Could you check a few things on this model? Use its own coordinates, in mm. Face numbers are marked on the shaded views. A direction names the side the tool comes from. Round coordinates to 2 decimals unless told otherwise and drop trailing zeros. Loops run counter-clockwise (first coordinate to the right, second up) from the corner with the lowest first, then second, coordinate; pieces in that order, holes last. Notation, with made-up numbers: M 44,-9.5 L 91,-9.5 A16 ccw 91,3.5 Z; hole C 18,18 d6. An arc over 180 degrees is marked long. Return JSON: item names as keys, results as strings. Group by question number.
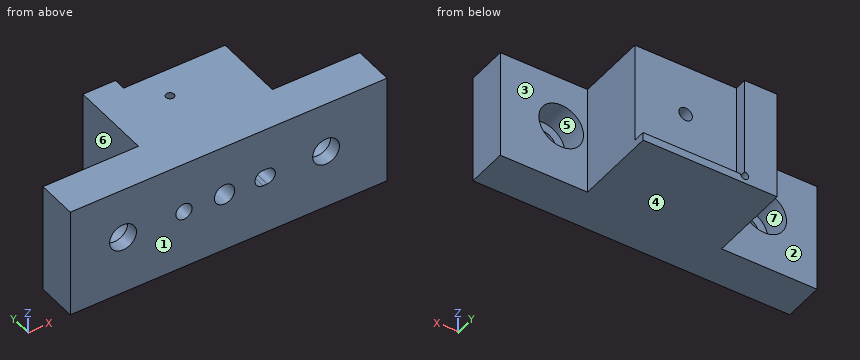
```python
from build123d import *

# Parameters (mm, degrees)
SKETCH_1_W                = 29
SKETCH_1_H                = 29
EXTRUDE_1_DEPTH           = 5
SKETCH_2_W                = 25
SKETCH_2_H                = 25
CUT_EXTRUDE_1_DEPTH       = 3
SKETCH_3_W                = 35
SKETCH_3_H                = 29
EXTRUDE_748_DEPTH         = 25.341167732
HOLE_WIZARD_M4_1_D        = 3.3
HOLE_WIZARD_M4_1_DEPTH    = 10.1
HOLE_WIZARD_M4_1_TIP      = 0.991420021
SKETCH_9_R                = 1
CUT_EXTRUDE_2_DEPTH       = 3
SKETCH_11_W               = 29
SKETCH_11_H               = 5
EXTRUDE_4_DEPTH           = 6
CUT_EXTRUDE_8_DEPTH       = 40.383835
SKETCH_19_W               = 80
SKETCH_19_H               = 25
EXTRUDE_5_DEPTH           = 10
HOLE_WIZARD_1_D           = 6.6
HOLE_WIZARD_1_DEPTH       = 10.1
HOLE_WIZARD_1_CBORE_D     = 11
HOLE_WIZARD_1_CBORE_DEPTH = 6.8
HOLE_WIZARD_1_TIP         = 1.982840043
SKETCH_23_W               = 80
SKETCH_23_H               = 10
EXTRUDE_6_DEPTH           = 2
SKETCH_24_W               = 27
SKETCH_24_H               = 10
CUT_EXTRUDE_9_DEPTH       = 2
MM_1_D                    = 4
MM_1_DEPTH                = 5
MM_1_TIP                  = 1.201721238
CUT_EXTRUDE_10_DEPTH      = 5
SKETCH_28_R               = 1
CUT_EXTRUDE_11_DEPTH      = 2
HOLE_WIZARD_M6_1_D        = 5
HOLE_WIZARD_M6_1_DEPTH    = 10
HOLE_WIZARD_M6_1_TIP      = 1.502151548


with BuildPart() as part:
    # 草图1 → 凸台-拉伸1 (new body)
    with BuildSketch(Plane(origin=(0, 0, 0), x_dir=(1, 0, 0), z_dir=(0, 1, 0))):
        Rectangle(SKETCH_1_W, SKETCH_1_H)
    extrude(amount=EXTRUDE_1_DEPTH)

    # 草图2 → 切除-拉伸1 (cut)
    with BuildSketch(Plane.XZ.offset(-5)):
        Rectangle(SKETCH_2_W, SKETCH_2_H)
    extrude(amount=CUT_EXTRUDE_1_DEPTH, mode=Mode.SUBTRACT)

    # 草图3 → Extrude 748 (add)
    with BuildSketch(Plane(origin=(0, 0, 0), x_dir=(-1, 0, 0), z_dir=(0, -1, 0))):
        with Locations((3, 0)):
            Rectangle(SKETCH_3_W, SKETCH_3_H)
    extrude(amount=EXTRUDE_748_DEPTH)

    # M4 螺纹孔1
    with Locations(Plane.ZX.offset(2)):
        with Locations((0, 0)):
            Hole(HOLE_WIZARD_M4_1_D / 2, depth=HOLE_WIZARD_M4_1_DEPTH)
            with Locations((0, 0, -(HOLE_WIZARD_M4_1_DEPTH + HOLE_WIZARD_M4_1_TIP / 2))):  # 118° drill point
                Cone(0, HOLE_WIZARD_M4_1_D / 2, HOLE_WIZARD_M4_1_TIP, mode=Mode.SUBTRACT)

    # 草图9 → 切除-拉伸2 (cut)
    with BuildSketch(Plane(origin=(0, 5, 0), x_dir=(1, 0, 0), z_dir=(0, 1, 0))):
        with Locations((-12.5, 12.5)):
            Circle(SKETCH_9_R)
    extrude(amount=-CUT_EXTRUDE_2_DEPTH, mode=Mode.SUBTRACT)

    # 草图11 → 凸台-拉伸4 (add)
    with BuildSketch(Plane.ZY.offset(14.5)):
        with Locations((0, 2.5)):
            Rectangle(SKETCH_11_W, SKETCH_11_H)
    extrude(amount=EXTRUDE_4_DEPTH)

    # 草图17 → 切除-拉伸8 (cut, through all)
    with BuildSketch(Plane(origin=(0, 5, 0), x_dir=(1, 0, 0), z_dir=(0, 1, 0))):
        Polygon((-20.5, -14.5), (14.5, -14.5), (14.5, 14.5), (12.5, 14.5), (12.5, -12.5), (-20.5, -12.5), align=None)
    extrude(amount=-CUT_EXTRUDE_8_DEPTH, mode=Mode.SUBTRACT)

    # 草图19 → 凸台-拉伸5 (add)
    with BuildSketch(Plane(origin=(0, -25.341167732, 0), x_dir=(-1, 0, 0), z_dir=(0, -1, 0))):
        with Locations((6, 0)):
            Rectangle(SKETCH_19_W, SKETCH_19_H)
    extrude(amount=-EXTRUDE_5_DEPTH)

    # 打孔尺寸(%根据)内六角圆柱头螺钉的类型1
    with Locations(Plane(origin=(-31, -15.341167732, 0), x_dir=(0, 0, 1), z_dir=(0, 1, 0))):
        with Locations((0, 0), (0, 50)):
            CounterBoreHole(HOLE_WIZARD_1_D / 2, HOLE_WIZARD_1_CBORE_D / 2, HOLE_WIZARD_1_CBORE_DEPTH, depth=HOLE_WIZARD_1_DEPTH)
            with Locations((0, 0, -(HOLE_WIZARD_1_DEPTH + HOLE_WIZARD_1_TIP / 2))):  # 118° drill point
                Cone(0, HOLE_WIZARD_1_D / 2, HOLE_WIZARD_1_TIP, mode=Mode.SUBTRACT)

    # 草图23 → 凸台-拉伸6 (add)
    with BuildSketch(Plane(origin=(0, 0, -12.5), x_dir=(-1, 0, 0), z_dir=(0, 0, -1))):
        with Locations((6, -20.341167732)):
            Rectangle(SKETCH_23_W, SKETCH_23_H)
    extrude(amount=EXTRUDE_6_DEPTH)

    # 草图24 → 切除-拉伸9 (cut)
    with BuildSketch(Plane.ZY.offset(46)):
        with Locations((-1, -20.341167732)):
            Rectangle(SKETCH_24_W, SKETCH_24_H)
    extrude(amount=-CUT_EXTRUDE_9_DEPTH, mode=Mode.SUBTRACT)

    # 大小mm 暗销孔1
    with Locations(Plane(origin=(-16, -25.341167732, 0), x_dir=(0, 0, -1), z_dir=(0, -1, 0))):
        with Locations((0, 0)):
            Hole(MM_1_D / 2, depth=MM_1_DEPTH)
            with Locations((0, 0, -(MM_1_DEPTH + MM_1_TIP / 2))):  # 118° drill point
                Cone(0, MM_1_D / 2, MM_1_TIP, mode=Mode.SUBTRACT)

    # 草图27 → 切除-拉伸10 (cut)
    with BuildSketch(Plane.XZ.offset(25.341167732)):
        with BuildLine():
            Line((3.5, 2), (4.5, 2))
            ThreePointArc((4.5, 2), (6.5, 0), (4.5, -2))
            Line((4.5, -2), (3.5, -2))
            ThreePointArc((3.5, -2), (1.5, 0), (3.5, 2))
        make_face()
    extrude(amount=-CUT_EXTRUDE_10_DEPTH, mode=Mode.SUBTRACT)

    # 草图28 → 切除-拉伸11 (cut)
    with BuildSketch(Plane.XY.offset(12.5)):
        with Locations((-6, -5.341167732)):
            Circle(SKETCH_28_R)
    extrude(amount=-CUT_EXTRUDE_11_DEPTH, mode=Mode.SUBTRACT)

    # M6 螺纹孔1
    with Locations(Plane(origin=(-6, -25.341167732, 0), x_dir=(0, 0, -1), z_dir=(0, -1, 0))):
        with Locations((0, 0)):
            Hole(HOLE_WIZARD_M6_1_D / 2, depth=HOLE_WIZARD_M6_1_DEPTH)
            with Locations((0, 0, -(HOLE_WIZARD_M6_1_DEPTH + HOLE_WIZARD_M6_1_TIP / 2))):  # 118° drill point
                Cone(0, HOLE_WIZARD_M6_1_D / 2, HOLE_WIZARD_M6_1_TIP, mode=Mode.SUBTRACT)


solid = part.part
```
1. I need wall thicknesses on probe 1 along X at (y, z) = (-16.75, 0); probe 2 along X at (y, z) = (-24.55, 0); probe 3 along Y at (x, z) = (21.5, 6.25). Which ranges of each line are inside material? Lowest first, please.
2. We'd pull the mould along Z, two halves only. Please class the marked faces 4, 5, 6 and 7: +Z half, -Z half, draft (parallel to the pull), parting line (faces both ways), or undercut.
3. If we section it at B-B, the plane z = 6.75: Please give me the cut outline in (x, y).
4. I'm going to push flat-ended pins straight in: pin 1 Ø10 at (y, z) = (-4.5, -5) entering from -X; pin 2 Ø9 at (x, z) = (-31, 0) entering from +Y; pin 3 Ø12 at (y, z) = (-9.5, 2) entering from -X; pin 4 Ø1.2 at (x, z) = (-12.5, -12.5) entering from +Y. Where does each tip first touch, or does it pass through?
5. If we section it at A-A, the plane y = 1: Please give me the cut outline in (x, z), then the cut area to 3 significant figures.
6. If we section it at C-C, the plane x = 2.5: Please give me the cut outline in (y, z), then the cut area to 3 significant figures.
7. On a 3-axis mill with a long thin cutter (end or side, diameter ignored), from which of +Z, -Z, +X, -X, +Y, -Y can I reach the whole of each face in a straight line? I mean the marked faces 1, 2 and 3. Say none if no direction works.
8. If we section it at D-D, the plane y = -11: Please give me the cut outline in (x, z).
Geometry results:
{
 "1": {"probe 1": "-44 to -36.5, -25.5 to -8.5, -3.5 to 13.5, 24.5 to 34", "probe 2": "-44 to -34.3, -27.7 to -18, -14 to -8.5, -3.5 to 1.5, 6.5 to 15.7, 22.3 to 34", "probe 3": "-25.34 to -15.34"},
 "2": {"face 4": "-Z half", "face 5": "undercut", "face 6": "draft", "face 7": "undercut"},
 "3": {"outline": "M -44,-25.34 L 34,-25.34 L 34,-15.34 L 12.5,-15.34 L 12.5,2 L -12.5,2 L -12.5,5 L -20.5,5 L -20.5,-15.34 L -44,-15.34 Z"},
 "4": {"pin 1": "x = -20.5", "pin 2": "y = -22.14", "pin 3": "x = -44", "pin 4": "y = 2"},
 "5": {"outline": "M -20.5,-14.5 L 12.5,-14.5 L 12.5,12.5 L -20.5,12.5 Z; hole C 0,0 d3.3", "area": "882 mm^2"},
 "6": {"outline": "M -25.34,-14.5 L 5,-14.5 L 5,-12.5 L 2,-12.5 L 2,12.5 L -25.34,12.5 L -25.34,1.73 L -20.34,1.73 L -20.34,-1.73 L -25.34,-1.73 Z", "area": "727 mm^2"},
 "7": {"face 1": "+Z, -Z, +X, -X, -Y", "face 2": "+Z, -Z, -X, +Y", "face 3": "+Z, -Z, +X, +Y"},
 "8": {"outline": "M -20.5,-14.5 L 12.5,-14.5 L 12.5,12.5 L -20.5,12.5 Z"}
}
